Could you check a few things on this model? Use its own coordinates, in mm. Face numbers are marked on the shaded views. A direction names the side the tool comes from. Give positions to 0.01 mm unless a question says otherwise; leave off trailing zeros. Write each loop counter-clockwise with the first axis right and the second up, starting at its lowest first coordinate (ties: lowest second). Pieces come first, ordered by that corner, then holes. Notation, with made-up numbers: (29, -34) -> (42, -34) arc R16 cw to (42, -14) -> close; hole circle Ø11 at (-38, 31.25). An arc over 180 degrees is marked (long way). One line per question, with ' | ' between items.
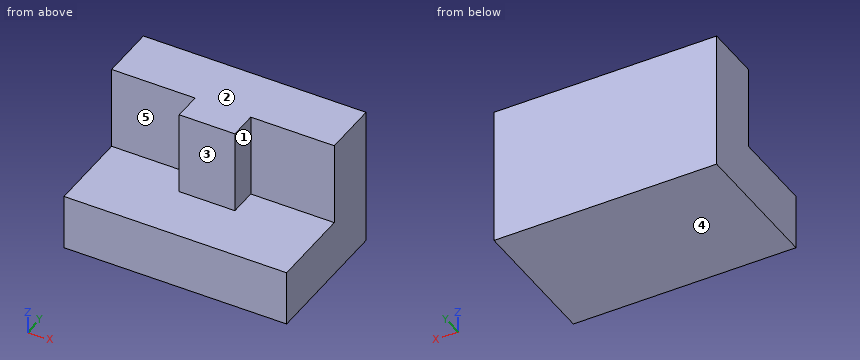
from build123d import *

# Parameters (mm, degrees)
F0_W     = 50.8
F0_H     = 31.75
F1_DEPTH = 31.75
F2_W     = 19.05
F2_H     = 19.05
F3_DEPTH = 19.05
F4_W     = 19.05
F4_H     = 19.05
F5_DEPTH = 19.05
F6_W     = 12.7
F6_H     = 19.05
F7_DEPTH = 12.7


with BuildPart() as f1:
    # F0 (on Front) → F1 (new body)
    with BuildSketch(Plane.XZ):
        with Locations((34.053563, 18.300161)):
            Rectangle(F0_W, F0_H)
    extrude(amount=F1_DEPTH)

    # F2 (on face) → F3 (cut)
    with BuildSketch(Plane.XZ.offset(31.75)):
        with Locations((18.178563, 24.650161)):
            Rectangle(F2_W, F2_H)
    extrude(amount=-F3_DEPTH, mode=Mode.SUBTRACT)

    # F4 (on face) → F5 (cut)
    with BuildSketch(Plane.XZ.offset(31.75)):
        with Locations((49.928563, 24.650161)):
            Rectangle(F4_W, F4_H)
    extrude(amount=-F5_DEPTH, mode=Mode.SUBTRACT)

    # F6 (on face) → F7 (cut)
    with BuildSketch(Plane.XZ.offset(31.75)):
        with Locations((34.053563, 24.650161)):
            Rectangle(F6_W, F6_H)
    extrude(amount=-F7_DEPTH, mode=Mode.SUBTRACT)


solid = f1.part
Q1. Imagine slicing it at D-D on x = 23. Please give me the cut outline in (y, z).
Answer below:
outline: (-31.75, 2.43) -> (0, 2.43) -> (0, 34.18) -> (-12.7, 34.18) -> (-12.7, 15.13) -> (-31.75, 15.13) -> close
Q2. Will these pins go through, and if not, where does the flat tip stop? pin 1 (5.5 mm diameter, centred on x = 20.5, z = 23, fed in from -Y); pin 2 (10 mm diameter, centred on x = 32.5, z = 30.5, fed in from -Y); pin 3 (7 mm diameter, centred on y = -16.5, z = 27, fed in from +X).
Answer below:
pin 1: stops at y = -12.7 | pin 2: stops at y = -19.05 | pin 3: stops at x = 40.4
Q3. On a 3-axis mill with a long thin cutter (end or side, diameter ignored), from which of +Z, -Z, +X, -X, +Y, -Y can I reach the whole of each face in a straight line? I mean the marked faces 1, 2, 3, 4 and 5. Say none if no direction works.
Answer below:
face 1: +Z, +X, -Y | face 2: +Z, +X, -X, +Y, -Y | face 3: +Z, +X, -X, -Y | face 4: -Z, +X, -X, +Y, -Y | face 5: +Z, -X, -Y
Q4. If I drill on line 1 along Z through (x, y) = (51.5, -18); line 2 along Y through (x, z) = (44.5, 24); line 3 along Y through (x, z) = (37, 28), over which ranges is the centre line in solid material (lowest first)?
Answer below:
line 1: z = 2.43 to 15.13 | line 2: y = -12.7 to 0 | line 3: y = -19.05 to 0
Q5. Imagine slicing it at A-A on y = -18.5. Please give me the cut outline in (x, z), and give its area (3 significant figures).
Answer below:
outline: (8.65, 2.43) -> (59.45, 2.43) -> (59.45, 15.13) -> (40.4, 15.13) -> (40.4, 34.18) -> (27.7, 34.18) -> (27.7, 15.13) -> (8.65, 15.13) -> close | area: 887 mm^2
Q6. Imagine slicing it at C-C on x = 34.5. Please give me the cut outline in (y, z).
Answer below:
outline: (-31.75, 2.43) -> (0, 2.43) -> (0, 34.18) -> (-19.05, 34.18) -> (-19.05, 15.13) -> (-31.75, 15.13) -> close
Q7. Imagine slicing it at B-B on z = 19.5. Please give me the cut outline in (x, y).
Answer below:
outline: (8.65, -12.7) -> (27.7, -12.7) -> (27.7, -19.05) -> (40.4, -19.05) -> (40.4, -12.7) -> (59.45, -12.7) -> (59.45, 0) -> (8.65, 0) -> close
